Source: CAD feature listing. Evaluate the final solid. Frame: model axes, mm. Face numbers are marked on the shaded views. A direction names the side the tool comes from. Coordinates: 2 decimals unless noted, no trailing zeros. Loops run counter-clockwise (first coordinate to the right, second up) from the corner with the lowest first, then second, coordinate; pieces in that order, holes last. Notation, with made-up numbers: M 53,18 L 100,18 A17 cw 100,48 Z; hole C -34.5,75.25 d10. An arc over 180 degrees is marked long. One line per question, with ' | ' between items. Start each with the question number.
1. Ray query, probe 1 along X at (y, z) = (-3.5, 26.5); probe 2 along X at (y, z) = (-6, 12); probe 3 along Z at (x, y) = (-12, -2). Return the intervals inside material, ascending.
2. Section query C-C, the plane z = 3. Output: boundary loops of the cut face in (x, y) (3 decimals), and give its area (3 significant figures).
3. Access query for the marked faces 4, 5 and 6. Directions: +Z, -Z, +X, -X, +Y, -Y. A direction counts if a zero-diameter tool reaches every point of the face in a straight line with its end or side. Return the directions, or none.
4. Section query D-D, the plane y = -10. Output: boundary loops of the cut face in (x, z).
5. Section query A-A, the plane z = 22.5. Output: boundary loops of the cut face in (x, y), and give its area (3 significant figures).
6. Mould query, pull axis Z, two halves, no side actions, for the marked faces 1, 2 and 3. Classes: pulls with the +Z half, pulls with the -Z half, needs draft (parallel to the pull), parting line crosses it, or undercut.
7. Pin query (flat end, axial travel): P1, Ø2, axis at x = 0.5, z = 8, coming from the +Y side; P2, Ø10, axis at x = -11.5, z = 18, coming from the -Y side; P3, Ø10, axis at x = 6, y = -2, coming from the -Z side; P4, Ø3, axis at x = 3, z = 29.5, coming from the +Y side. Return the tip coordinate at first contact, or that it passes through.
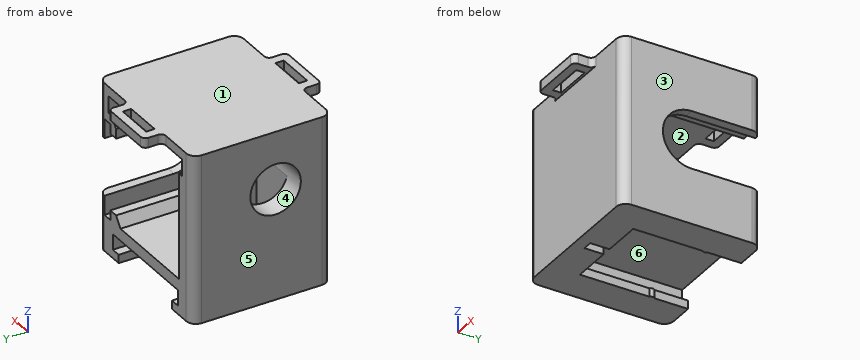
```python
from build123d import *

# Parameters (mm, degrees)
SKETCH1_W                         = 32
SKETCH1_H                         = 29
BOSS_EXTRUDE1_DEPTH               = 35
FILLET1_R                         = 2
SLOT_FOR_COIL_DEPTH               = 1
SLOT_FOR_COIL_DEPTH_BACK          = 30
BOSS_EXTRUDE2_DEPTH               = 6.5
BOSS_EXTRUDE3_DEPTH               = 1.75
SKETCH5_W                         = 2
SKETCH5_H                         = 6.5
SLOT_TO_FEED_IN_WIRE_DEPTH        = 33
SLOT_FO_PCB_DEPTH                 = 22.5
SKETCH7_W                         = 2
SKETCH7_H                         = 33
BOSS_EXTRUDE4_DEPTH               = 2.5
FILLET2_R                         = 6
ROD_MOUNT_SLOT_REACH              = 34
SKETCH14_W                        = 2.5
SKETCH14_H                        = 20
SIDE_CAVITY_FOR_MOUNT_PLATE_DEPTH = 22.5
SKETCH16_W                        = 2
SKETCH16_H                        = 2
SIDE_STOPS_FOR_MOUNT_PLATE_DEPTH  = 22.5
BOSS_EXTRUDE6_DEPTH               = 22.5
SKETCH21_W                        = 12
SKETCH21_H                        = 2
BOSS_EXTRUDE7_DEPTH               = 4
SKETCH23_W                        = 8
SKETCH23_H                        = 1.75
CUT_EXTRUDE7_DEPTH                = 2
FILLET3_R                         = 1
CUT_EXTRUDE8_REACH                = 34
SKETCH26_R                        = 5.25


with BuildPart() as part:
    # Sketch1 → Boss-Extrude1 (new body)
    with BuildSketch(Plane.XY):
        Rectangle(SKETCH1_W, SKETCH1_H)
    extrude(amount=BOSS_EXTRUDE1_DEPTH)

    # Fillet1
    fillet1_edges = [part.edges().sort_by_distance(p)[0] for p in [
        (16, -14.5, 17.5),
        (-16, -14.5, 17.5),
        (-16, 14.5, 17.5),
        (16, 14.5, 17.5),
    ]]
    fillet(fillet1_edges, radius=FILLET1_R)

    # Sketch2 → Slot for Coil (cut, two sides)
    with BuildSketch(Plane.XZ.offset(14.5)) as slot_for_coil_sk:
        Polygon((-9.125, 0), (-9.125, 1.75), (-11.125, 1.75), (-11.125, 5), (11.125, 5), (11.125, 1.75), (9.125, 1.75), (9.125, 0), align=None)
    extrude(amount=SLOT_FOR_COIL_DEPTH, mode=Mode.SUBTRACT)
    extrude(slot_for_coil_sk.sketch, amount=-SLOT_FOR_COIL_DEPTH_BACK, mode=Mode.SUBTRACT)

    # Sketch3 → Boss-Extrude2 (add)
    with BuildSketch(Plane.XZ.offset(14.5)):
        Polygon((-9.125, 0), (-9.125, 1.75), (-11.125, 1.75), (-11.125, 5), (11.125, 5), (11.125, 1.75), (9.125, 1.75), (9.125, 0), align=None)
    extrude(amount=-BOSS_EXTRUDE2_DEPTH)

    # Sketch4 → Boss-Extrude3 (add)
    with BuildSketch(Plane(origin=(0, 0, 1.75), x_dir=(-1, 0, 0), z_dir=(0, 0, -1))):
        with BuildLine():
            Line((-9.125, 7.5), (-9.125, 6.5))
            ThreePointArc((-9.125, 6.5), (-8.875, 7), (-9.125, 7.5))
        make_face()
    boss_extrude3 = extrude(amount=BOSS_EXTRUDE3_DEPTH)

    # Mirror1: Boss-Extrude3 across plane
    add(boss_extrude3.mirror(Plane(origin=(0, 0, 0), x_dir=(0, 0, 1), z_dir=(1, 0, 0))))

    # Sketch5 → slot to feed in wire (cut)
    with BuildSketch(Plane(origin=(0, 0, 0), x_dir=(-1, 0, 0), z_dir=(0, 0, -1))):
        with Locations((0, -11.25)):
            Rectangle(SKETCH5_W, SKETCH5_H)
    extrude(amount=-SLOT_TO_FEED_IN_WIRE_DEPTH, mode=Mode.SUBTRACT)

    # Sketch6 → slot fo PCB (cut)
    with BuildSketch(Plane(origin=(0, 14.5, 0), x_dir=(1, 0, 0), z_dir=(0, 1, 0))):
        Polygon((11.5, -7.5), (-11.5, -7.5), (-11.5, -29.5), (-12.55, -29.5), (-12.55, -33), (12.55, -33), (12.55, -29.5), (11.5, -29.5), align=None)
    extrude(amount=-SLOT_FO_PCB_DEPTH, mode=Mode.SUBTRACT)

    # Sketch7 → Boss-Extrude4 (add)
    with BuildSketch(Plane.XZ.offset(14.5)):
        with Locations((0, 16.5)):
            Rectangle(SKETCH7_W, SKETCH7_H)
    extrude(amount=-BOSS_EXTRUDE4_DEPTH)

    # Fillet2
    fillet2_edges = [part.edges().sort_by_distance(p)[0] for p in [
        (0, -12, 33),
    ]]
    fillet(fillet2_edges, radius=FILLET2_R)

    # Sketch11 → Rod Mount Slot (cut, up to next)
    with BuildSketch(Plane(origin=(16, 0, 44), x_dir=(0, 0, -1), z_dir=(1, 0, 0)), mode=Mode.PRIVATE) as rod_mount_slot_sk1:
        with BuildLine():
            Line((32.5, 25), (32.5, 0))
            ThreePointArc((32.5, 0), (26.5, -6), (20.5, 0))
            Line((20.5, 0), (20.5, 25))
            ThreePointArc((20.5, 25), (26.5, 31), (32.5, 25))
        make_face()
    rod_mount_slot_tool1 = extrude(rod_mount_slot_sk1.sketch, amount=-ROD_MOUNT_SLOT_REACH, mode=Mode.PRIVATE) & part.part
    add(rod_mount_slot_tool1.solids().sort_by_distance((16, 12.5, 17.5))[0], mode=Mode.SUBTRACT)

    # Sketch14 → Side cavity for mount plate (cut)
    with BuildSketch(Plane(origin=(0, 14.5, 0), x_dir=(1, 0, 0), z_dir=(0, 1, 0))):
        with Locations((12.75, -17.5)):
            Rectangle(SKETCH14_W, SKETCH14_H)
    extrude(amount=-SIDE_CAVITY_FOR_MOUNT_PLATE_DEPTH, mode=Mode.SUBTRACT)

    # Sketch16 → Side stops for mount plate (add)
    with BuildSketch(Plane(origin=(0, 14.5, 0), x_dir=(1, 0, 0), z_dir=(0, 1, 0))):
        with Locations((11, -8.5)):
            Rectangle(SKETCH16_W, SKETCH16_H)
        with Locations((11, -26.5)):
            Rectangle(SKETCH16_W, SKETCH16_H)
    extrude(amount=-SIDE_STOPS_FOR_MOUNT_PLATE_DEPTH)

    # Sketch20 → Boss-Extrude6 (add)
    with BuildSketch(Plane(origin=(0, 14.5, 0), x_dir=(1, 0, 0), z_dir=(0, 1, 0))):
        Polygon((11.5, -29.5), (10, -27.5), (11.5, -27.5), align=None)
        Polygon((10, -9.5), (8.5, -7.5), (10, -7.5), align=None)
    extrude(amount=-BOSS_EXTRUDE6_DEPTH)

    # Sketch21 → Boss-Extrude7 (add)
    with BuildSketch(Plane(origin=(0, 14.5, 0), x_dir=(-1, 0, 0), z_dir=(0, 1, 0))):
        with Locations((0, 34)):
            Rectangle(SKETCH21_W, SKETCH21_H)
    boss_extrude7 = extrude(amount=BOSS_EXTRUDE7_DEPTH)

    # Sketch23 → Cut-Extrude7 (cut)
    with BuildSketch(Plane.XY.offset(35)):
        with Locations((0, 15.875)):
            Rectangle(SKETCH23_W, SKETCH23_H)
    cut_extrude7 = extrude(amount=-CUT_EXTRUDE7_DEPTH, mode=Mode.SUBTRACT)

    # Mirror3: Boss-Extrude7, Cut-Extrude7 across plane
    add(boss_extrude7.mirror(Plane.ZX))
    add(cut_extrude7.mirror(Plane.ZX), mode=Mode.SUBTRACT)

    # Fillet3
    fillet3_edges = [part.edges().sort_by_distance(p)[0] for p in [
        (6, 14.5, 34),
        (-6, 14.5, 34),
        (6, 18.5, 34),
        (-6, 18.5, 34),
        (6, -18.5, 34),
        (-6, -18.5, 34),
        (6, -14.5, 34),
        (-6, -14.5, 34),
    ]]
    fillet(fillet3_edges, radius=FILLET3_R)

    # Sketch26 → Cut-Extrude8 (cut, up to next)
    with BuildSketch(Plane(origin=(-16, 0, 0), x_dir=(0, 0, -1), z_dir=(1, 0, 0)), mode=Mode.PRIVATE) as cut_extrude8_sk1:
        with Locations((-23.015, -2.89)):
            Circle(SKETCH26_R)
    cut_extrude8_tool1 = extrude(cut_extrude8_sk1.sketch, amount=CUT_EXTRUDE8_REACH, mode=Mode.PRIVATE) & part.part
    add(cut_extrude8_tool1.solids().sort_by_distance((-16, -2.89, 23.015))[0], mode=Mode.SUBTRACT)


solid = part.part
```
Taken from the geometry:
1) probe 1: 10 to 12, 14 to 16 | probe 2: -16 to -11.5, 14 to 16 | probe 3: 0 to 17.84, 28.19 to 29.5, 33 to 35
2) outline: M -16,-12.5 A2 ccw -14,-14.5 L 14,-14.5 A2 ccw 16,-12.5 L 16,12.5 A2 ccw 14,14.5 L 11.125,14.5 L 11.125,-8 L 1,-8 L 1,-12 L -1,-12 L -1,-8 L -11.125,-8 L -11.125,14.5 L -14,14.5 A2 ccw -16,12.5 Z | area: 416 mm^2
3) face 4: -X | face 5: +Z, -Z, -X, +Y, -Y | face 6: +Y
4) outline: M -16,0 L -1,0 L -1,31.47 L 1,31.47 L 1,0 L 16,0 L 16,35 L -16,35 Z
5) outline: M -16,-12.5 A2 ccw -14,-14.5 L 14,-14.5 A2 ccw 16,-12.5 L 16,-3.32 L 14,-3.32 L 14,-8 L 1,-8 L 1,-12 L -1,-12 L -1,-8.11 L -16,-8.11 Z; M -16,2.33 L -11.5,2.33 L -11.5,14.5 L -14,14.5 A2 ccw -16,12.5 Z | area: 260 mm^2
6) face 1: pulls with the +Z half | face 2: undercut | face 3: needs draft
7) P1: y = 14.5 | P2: y = -14.5 | P3: z = 0 | P4: y = -8
